Read the model definition and answer for the solid it produces. Units are mm, in the model's axes. A direction names the side the tool comes from. Coordinates: 2 decimals unless noted, no trailing zeros. Write each loop counter-clockwise with the first axis right and the second up, starting at its lowest first coordinate (ties: lowest second). Pieces come first, ordered by that corner, then holes.
(1) Given pin 1 (3.5 mm diameter, centred on x = -14, y = -12.26, fed in from +Z); pin 2 (1.5 mm diameter, centred on y = 15, z = 0.5, fed in from +X); pin 3 (1.3 mm diameter, centred on x = -1.5, z = 1.5, fed in from -Y); pin 4 (1 mm diameter, centred on y = -8.5, z = 0.5, fed in from +X), each flat-ended and moving along its own axis, determine where each tip first touches the part or whether it passes through.
(2) Find the intervals of material crossed by probe 1 along Y at (x, z) = (-14, 2.2); probe 2 along Y at (x, z) = (-4, 3.95); probe 3 along Y at (x, z) = (-18, 0.7), in increasing order.
(3) Which of the six approach directions +Z, -Z, +X, -X, +Y, -Y give full straight-line access (tool end or side, diameter ignored) to faces 5 (the flat face through (8.32, -11.61, 2.07)), 6 (the flat face through (0, 4, 0))?
(4) The mould has two halves that part along Y. Classify faces 1 (the flat face through (0, 4, 4.2)), 2 (the cylindrical face through (17.279, 15.615, 2.071)), 3 (the flat face through (15, -15.566, 2)), 4 (the flat face through (0, 23.255, 2)): +Y half, -Y half, draft (parallel to the pull), parting line (faces both ways), or undercut.
(5) Section C-C on x = 2 is taken. Write down the section's boundary in (y, z), then the cut area to 3 significant figures.
(6) Section B-B on z = 0.85 is taken. Write down the section's boundary in (x, y), then the cut area to 3 significant figures.
(7) Section A-A on x = -14 is taken. Write down the section's boundary in (y, z), then the cut area to 3 significant figures.
(8) Section D-D on x = 18 is taken. Write down the section's boundary in (y, z), then the cut area to 3 significant figures.
from build123d import *

# Parameters (mm, degrees)
F0_R     = 2.061288
F0_R_2   = 2.172791
F1_DEPTH = 4.2


with BuildPart() as f1:
    # F0 (on Top) → F1 (new body)
    with BuildSketch(Plane.XY):
        with BuildLine():
            Line((16.011793, 23.255279), (0, 23.255279))
            Line((0, 23.255279), (-16.011793, 23.255279))
            ThreePointArc((-16.011793, 23.255279), (-20.363271, 21.386215), (-22.003686, 16.94349))
            Line((-22.003686, 16.94349), (-20.336709, -15.092083))
            ThreePointArc((-20.336709, -15.092083), (-20.181629, -15.428724), (-19.837385, -15.566101))
            Line((-19.837385, -15.566101), (-10.547646, -15.566101))
            ThreePointArc((-10.547646, -15.566101), (-10.282024, -15.48971), (-10.097566, -15.283881))
            Line((-10.097566, -15.283881), (-6.591564, -8.038143))
            ThreePointArc((-6.591564, -8.038143), (-6.407106, -7.832314), (-6.141484, -7.755924))
            Line((-6.141484, -7.755924), (0, -7.755924))
            Line((0, -7.755924), (6.141484, -7.755924))
            ThreePointArc((6.141484, -7.755924), (6.407106, -7.832314), (6.591564, -8.038143))
            Line((6.591564, -8.038143), (10.097566, -15.283881))
            ThreePointArc((10.097566, -15.283881), (10.282024, -15.48971), (10.547646, -15.566101))
            Line((10.547646, -15.566101), (19.837385, -15.566101))
            ThreePointArc((19.837385, -15.566101), (20.181629, -15.428724), (20.336709, -15.092083))
            Line((20.336709, -15.092083), (22.003686, 16.94349))
            ThreePointArc((22.003686, 16.94349), (20.363271, 21.386215), (16.011793, 23.255279))
        make_face()
        with Locations((-14, -12.264313)):
            Circle(F0_R, mode=Mode.SUBTRACT)
        with Locations((14, -12.264313)):
            Circle(F0_R, mode=Mode.SUBTRACT)
        with Locations((-17.75, 17.735687)):
            Circle(F0_R_2, mode=Mode.SUBTRACT)
        with Locations((17.75, 17.735687)):
            Circle(F0_R_2, mode=Mode.SUBTRACT)
    extrude(amount=F1_DEPTH)


solid = f1.part
Response:
1. pin 1: passes through
1. pin 2: stops at x = 21.94
1. pin 3: stops at y = -7.76
1. pin 4: stops at x = 20.71
2. probe 1: y = -15.57 to -14.33, -10.2 to 23.26
2. probe 2: y = -7.76 to 23.26
2. probe 3: y = -15.57 to 15.58, 19.89 to 22.92
3. face 5: +Z, -Z, -Y
3. face 6: -Z, +X, -X, +Y, -Y
4. face 1: draft
4. face 2: undercut
4. face 3: -Y half
4. face 4: +Y half
5. outline: (-7.76, 0) - (23.26, 0) - (23.26, 4.2) - (-7.76, 4.2) - close
5. area: 130 mm2
6. outline: (-22, 16.94) - (-20.34, -15.09) arc R0.5 ccw to (-19.84, -15.57) - (-10.55, -15.57) arc R0.5 ccw to (-10.1, -15.28) - (-6.59, -8.04) arc R0.5 cw to (-6.14, -7.76) - (6.14, -7.76) arc R0.5 cw to (6.59, -8.04) - (10.1, -15.28) arc R0.5 ccw to (10.55, -15.57) - (19.84, -15.57) arc R0.5 ccw to (20.34, -15.09) - (22, 16.94) arc R6 ccw to (16.01, 23.26) - (-16.01, 23.26) arc R6 ccw to start; hole circle Ø4.35 at (-17.75, 17.74); hole circle Ø4.12 at (-14, -12.26); hole circle Ø4.12 at (14, -12.26); hole circle Ø4.35 at (17.75, 17.74)
6. area: 1,450 mm2
7. outline: (-15.57, 0) - (-14.33, 0) - (-14.33, 4.2) - (-15.57, 4.2) - close; (-10.2, 0) - (23.26, 0) - (23.26, 4.2) - (-10.2, 4.2) - close
7. area: 146 mm2
8. outline: (-15.57, 0) - (15.58, 0) - (15.58, 4.2) - (-15.57, 4.2) - close; (19.89, 0) - (22.92, 0) - (22.92, 4.2) - (19.89, 4.2) - close
8. area: 143 mm2
